Read the model definition and answer for the solid it produces. Units are mm, in the model's axes. Round coordinates to 2 decimals unless told otherwise and drop trailing zeros. Loops run counter-clockwise (first coordinate to the right, second up) from the corner with the lowest first, then second, coordinate; pieces in that order, holes last. Notation, with made-up numbers: (77.25, 64.5) -> (88.25, 64.5) arc R16 cw to (88.25, 94.5) -> close; hole circle Ø5 at (33.25, 11.25). An arc over 180 degrees is marked (long way). Put each result on its own line as item: value.
from build123d import *

# Parameters (mm, degrees)
F0_R     = 15
F0_R_2   = 9
F0_R_3   = 6
F0_R_4   = 2
F1_DEPTH = 4
F2_DEPTH = 20
F3_SIZE  = 1
F4_SIZE  = 2


with BuildPart() as f1:
    # F0 (on Top) → F1 (new body)
    with BuildSketch(Plane.XY):
        Circle(F0_R)
        Circle(F0_R_2, mode=Mode.SUBTRACT)
        Circle(F0_R_2)
        Circle(F0_R_3, mode=Mode.SUBTRACT)
        Circle(F0_R_3)
        Circle(F0_R_4, mode=Mode.SUBTRACT)
    extrude(amount=-F1_DEPTH)

    # F0 (on Top) → F2 (join)
    with BuildSketch(Plane.XY):
        Circle(F0_R_2)
        Circle(F0_R_3, mode=Mode.SUBTRACT)
    extrude(amount=F2_DEPTH)

    # F3
    f3_edges = [f1.edges().sort_by_distance(p)[0] for p in [
        (-2, 0, 0),
    ]]
    chamfer(f3_edges, length=F3_SIZE)

    # F4
    f4_edges = [f1.edges().sort_by_distance(p)[0] for p in [
        (-6, 0, 20),
    ]]
    chamfer(f4_edges, length=F4_SIZE)


solid = f1.part
Item 1: For a pull along X with two mould halves and no side action, classify faces 1 (the cylindrical face through (-6, 0, 9)), 2 (the cylindrical face through (0, -2, -2)), 3 (the flat face through (3, 0, -4)), 4 (the cylindrical face through (-14.985, 0.66, -1.972)) as pulls with the +X half, pulls with the -X half, needs draft (parallel to the pull), parting line crosses it, or undercut.
Derived:
face 1: undercut
face 2: undercut
face 3: needs draft
face 4: parting line crosses it
Item 2: The part is cut by section C-C (z = 15.75). Determine the outline of the cut face in (x, y).
Derived:
outline: circle Ø18 at (0, 0); hole circle Ø12 at (0, 0)
Item 3: Flat-ended cylindrical pins translate along their axes: pin 1 Ø6 at (y, z) = (7, -0.5) entering from -X; pin 2 Ø14 at (x, y) = (0, 0) entering from +Z; pin 3 Ø5 at (x, z) = (-1.5, 2) entering from -Y; pin 4 Ø9.5 at (x, y) = (-1.5, -2) entering from +Z. Find the tip coordinate at first contact, or state that the pin passes through.
Derived:
pin 1: stops at x = -14.46
pin 2: stops at z = 19
pin 3: stops at y = -15
pin 4: stops at z = 19.25
Item 4: Find the intervals of material crossed by line 1 along Y through (x, z) = (0, -1.8); line 2 along Y through (x, z) = (0, 10.75); line 3 along X through (y, z) = (-3.75, 13), in increasing order.
Derived:
line 1: y = -15 to -2, 2 to 15
line 2: y = -9 to -6, 6 to 9
line 3: x = -8.18 to -4.68, 4.68 to 8.18
Item 5: The part is cut by section A-A (y = 0). Determine the outline of the cut face in (x, z).
Derived:
outline: (-15, -4) -> (-2, -4) -> (-2, -1) -> (-3, 0) -> (-6, 0) -> (-6, 18) -> (-8, 20) -> (-9, 20) -> (-9, 0) -> (-15, 0) -> close; (2, -4) -> (15, -4) -> (15, 0) -> (9, 0) -> (9, 20) -> (8, 20) -> (6, 18) -> (6, 0) -> (3, 0) -> (2, -1) -> close
Item 6: The part is cut by section D-D (x = 8.5). Determine the outline of the cut face in (y, z), then the cut area to 3 significant figures.
Derived:
outline: (-12.36, -4) -> (12.36, -4) -> (12.36, 0) -> (2.96, 0) -> (2.96, 20) -> (-2.96, 20) -> (-2.96, 0) -> (-12.36, 0) -> close
area: 217 mm^2
